from build123d import *

# Parameters (mm, degrees)
ESTRUSIONE_ESTRUSIONE1_DEPTH                         = 170
FORO_LAMATO_PER_BULLONE_M5_A_TESTA_ESAGO_D           = 4.5
FORO_LAMATO_PER_BULLONE_M5_A_TESTA_ESAGO_DEPTH       = 30
FORO_LAMATO_PER_BULLONE_M5_A_TESTA_ESAGO_CBORE_D     = 10
FORO_LAMATO_PER_BULLONE_M5_A_TESTA_ESAGO_CBORE_DEPTH = 3
FORO_LAMATO_PER_BULLONE_M5_A_TESTA_ESAGO_TIP         = 1.351936393
SCHIZZO4_W                                           = 89
SCHIZZO4_H                                           = 35
TAGLIO_ESTRUSIONE1_DEPTH                             = 170
RACCORDO1_R                                          = 6


with BuildPart() as part:
    # Schizzo1 → Estrusione-Estrusione1 (new body)
    with BuildSketch(Plane(origin=(0, 0, 0), x_dir=(0, 0, -1), z_dir=(1, 0, 0))):
        with BuildLine():
            Line((0, 0), (6, 0))
            Line((6, 0), (6, 35))
            ThreePointArc((6, 35), (6.585786438, 36.414213562), (8, 37))
            Line((8, 37), (12, 37))
            ThreePointArc((12, 37), (14.828427125, 38.171572875), (16, 41))
            Line((16, 41), (16, 65))
            Line((16, 65), (10, 65))
            Line((10, 65), (10, 45))
            ThreePointArc((10, 45), (9.414213562, 43.585786438), (8, 43))
            Line((8, 43), (5, 43))
            ThreePointArc((5, 43), (1.464466094, 41.535533906), (0, 38))
            Line((0, 38), (0, 0))
        make_face()
    extrude(amount=ESTRUSIONE_ESTRUSIONE1_DEPTH)

    # Foro lamato per Bullone M5 a testa esagonale-1
    with Locations(Plane(origin=(0, 0, -6), x_dir=(-1, 0, 0), z_dir=(0, 0, -1))):
        with Locations((-25, 19.5), (-71, 19.5)):
            CounterBoreHole(FORO_LAMATO_PER_BULLONE_M5_A_TESTA_ESAGO_D / 2, FORO_LAMATO_PER_BULLONE_M5_A_TESTA_ESAGO_CBORE_D / 2, FORO_LAMATO_PER_BULLONE_M5_A_TESTA_ESAGO_CBORE_DEPTH, depth=FORO_LAMATO_PER_BULLONE_M5_A_TESTA_ESAGO_DEPTH)
            with Locations((0, 0, -(FORO_LAMATO_PER_BULLONE_M5_A_TESTA_ESAGO_DEPTH + FORO_LAMATO_PER_BULLONE_M5_A_TESTA_ESAGO_TIP / 2))):  # 118° drill point
                Cone(0, FORO_LAMATO_PER_BULLONE_M5_A_TESTA_ESAGO_D / 2, FORO_LAMATO_PER_BULLONE_M5_A_TESTA_ESAGO_TIP, mode=Mode.SUBTRACT)

    # Schizzo4 → Taglio-Estrusione1 (cut)
    with BuildSketch(Plane(origin=(0, 0, -6), x_dir=(-1, 0, 0), z_dir=(0, 0, -1))):
        with Locations((-125.5, 17.5)):
            Rectangle(SCHIZZO4_W, SCHIZZO4_H)
    extrude(amount=-TAGLIO_ESTRUSIONE1_DEPTH, mode=Mode.SUBTRACT)

    # Raccordo1
    raccordo1_edges = [part.edges().sort_by_distance(p)[0] for p in [
        (81, 35, -3),
    ]]
    fillet(raccordo1_edges, radius=RACCORDO1_R)


solid = part.part
Source: CAD feature listing. Evaluate the final solid. Frame: model axes, mm. A direction names the side the tool comes from. Coordinates: 2 decimals unless noted, no trailing zeros. Loops run counter-clockwise (first coordinate to the right, second up) from the corner with the lowest first, then second, coordinate; pieces in that order, holes last. Notation, with made-up numbers: (-14, 64.5) - (-6, 64.5) arc R31 cw to (-6, 92.5) - close; hole circle Ø11 at (-2, 2). An arc over 180 degrees is marked (long way). One line per item, written item: value. Start each with the question number.
1. Mould query, pull axis Y, two halves, no side actions, for faces 1 (the cylindrical face through (66.381, 17.585, -4.521)), 2 (the flat face through (84, 37, -10)), 3 (the cylindrical face through (29, 16.5, -4.5)), 4 (the flat face through (84, 55, -10)). Classes: pulls with the +Y half, pulls with the -Y half, needs draft (parallel to the pull), parting line crosses it, or undercut.
2. Ray query, L1, parallel to Y at x = 71, z = -5.3; L2, parallel to Z at x = 122, y = 54; L3, parallel to Z at x = 69, y = 10. Return the intervals inside material, ascending.
3. Section D-D (y = 11.5). Return the cut outline in (x, z), and give its area (3 significant figures).
4. Section C-C (x = 31.5). Return the cut outline in (y, z), and give its area (3 significant figures).
5. Section B-B (x = 71). Return the cut outline in (y, z), and give its area (3 significant figures).
6. Section A-A (y = 19.5). Return the cut outline in (x, z).
7. Set-up query: faces 5 (the flat face through (84, 43, -7)), 6 (the flat face through (43, 17, -6)), 7 (the flat face through (81, 14, -3)), 8 (the flat face through (24, 17, -3)), 9 (the flat face through (84, 65, -13)). Return all of +Z, -Z, +X, -X, +Y, -Y with unobstructed straight access to the full face (end or side cutting, diameter ignored); none if empty.
8. Contact query for flat-ended pins moving along their axis: P1, Ø9, axis at x = 71, y = 19.5, coming from the -Z side; P2, Ø6, axis at y = 21, z = -4.5, coming from the +X side; P3, Ø5, axis at x = 108.5, z = -3.5, coming from the -Y side. Output: stop coordinate, or through.
Verdict:
1. face 1: undercut
1. face 2: pulls with the -Y half
1. face 3: undercut
1. face 4: needs draft
2. L1: y = 0 to 14.5, 24.5 to 43
2. L2: z = -16 to -10
2. L3: z = -6 to 0
3. outline: (0, -6) - (81, -6) - (81, 0) - (0, 0) - close
3. area: 486 mm2
4. outline: (0, -6) - (35, -6) arc R2 cw to (37, -8) - (37, -12) arc R4 ccw to (41, -16) - (65, -16) - (65, -10) - (45, -10) arc R2 cw to (43, -8) - (43, -5) arc R5 ccw to (38, 0) - (0, 0) - close
4. area: 443 mm2
5. outline: (0, -6) - (14.5, -6) - (14.5, -3) - (17.25, -3) - (17.25, 0) - (0, 0) - close; (21.75, -3) - (24.5, -3) - (24.5, -6) - (35, -6) arc R2 cw to (37, -8) - (37, -12) arc R4 ccw to (41, -16) - (65, -16) - (65, -10) - (45, -10) arc R2 cw to (43, -8) - (43, -5) arc R5 ccw to (38, 0) - (21.75, 0) - close
5. area: 399 mm2
6. outline: (0, -6) - (20, -6) - (20, -3) - (22.75, -3) - (22.75, 0) - (0, 0) - close; (27.25, -3) - (30, -3) - (30, -6) - (66, -6) - (66, -3) - (68.75, -3) - (68.75, 0) - (27.25, 0) - close; (73.25, -3) - (76, -3) - (76, -6) - (81, -6) - (81, 0) - (73.25, 0) - close
7. face 5: +Z, +X, -X, +Y
7. face 6: -Z, +X, -X, -Y
7. face 7: +Z, -Z, +X, -Y
7. face 8: -Z
7. face 9: +Z, -Z, +X, -X, +Y
8. P1: stops at z = -3
8. P2: stops at x = 81
8. P3: stops at y = 35
